The model under review builds one solid part; all positions refer to its coordinate system, in mm. Coordinates: 2 decimals unless noted, no trailing zeros. Write each loop counter-clockwise with the first axis right and the second up, starting at its lowest first coordinate (ties: lowest second). Pieces come first, ordered by that corner, then holes.
1) Add section C-C, the plane x = 31.75. State the section outline as (y, z) points (3 decimals), then the cut area to 3 significant figures.
2) Add section D-D, the plane z = 7. State the section outline as (x, y) points (3 decimals), then the cut area to 3 significant figures.
3) Add section B-B, the plane z = 20. State the section outline as (x, y) points (3 decimals).
4) Add section A-A, the plane z = 44.45. State the section outline as (x, y) points (3 decimals), then the cut area to 3 significant figures.
5) For line 1 (X direction, y = 2.5, z = 33.15); line 2 (X direction, y = 0.9, z = 44.45); line 3 (Z direction, x = 29, y = 0.4), list the stretches that pass through material, from the lowest coordinate up.
from build123d import *

# Parameters (mm, degrees)
SKETCH1_W          = 38.1
SKETCH1_H          = 50.8
SKETCH1_R          = 1.65
SKETCH1_R_2        = 7.5
SKETCH1_R_3        = 3.2639
BASE_EXTRUDE_DEPTH = 3.175


with BuildPart() as part:
    # Sketch1 → Base Extrude (new body)
    with BuildSketch(Plane(origin=(0, 0, 0), x_dir=(1, 0, 0), z_dir=(0, 1, 0))):
        with Locations((19.05, -25.4)):
            Rectangle(SKETCH1_W, SKETCH1_H)
        with Locations((19.05, -40.9)):
            Circle(SKETCH1_R, mode=Mode.SUBTRACT)
        with Locations((5.626606241, -33.15)):
            Circle(SKETCH1_R, mode=Mode.SUBTRACT)
        with Locations((5.626606241, -17.65)):
            Circle(SKETCH1_R, mode=Mode.SUBTRACT)
        with Locations((19.05, -9.9)):
            Circle(SKETCH1_R, mode=Mode.SUBTRACT)
        with Locations((32.473393759, -17.65)):
            Circle(SKETCH1_R, mode=Mode.SUBTRACT)
        with Locations((32.473393759, -33.15)):
            Circle(SKETCH1_R, mode=Mode.SUBTRACT)
        with Locations((19.05, -25.4)):
            Circle(SKETCH1_R_2, mode=Mode.SUBTRACT)
        with Locations((6.35, -6.35)):
            Circle(SKETCH1_R_3, mode=Mode.SUBTRACT)
        with Locations((31.75, -6.35)):
            Circle(SKETCH1_R_3, mode=Mode.SUBTRACT)
        with Locations((6.35, -44.45)):
            Circle(SKETCH1_R_3, mode=Mode.SUBTRACT)
        with Locations((31.75, -44.45)):
            Circle(SKETCH1_R_3, mode=Mode.SUBTRACT)
    extrude(amount=BASE_EXTRUDE_DEPTH)


solid = part.part
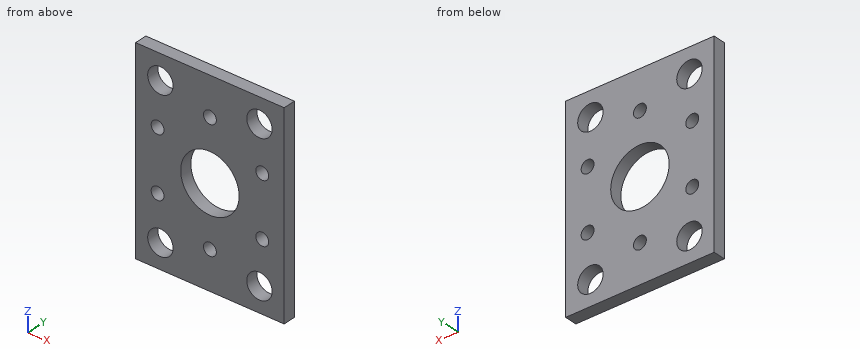
Geometry results:
1. outline: (0, 0) - (3.175, 0) - (3.175, 3.086) - (0, 3.086) - close; (0, 9.614) - (3.175, 9.614) - (3.175, 16.167) - (0, 16.167) - close; (0, 19.133) - (3.175, 19.133) - (3.175, 31.667) - (0, 31.667) - close; (0, 34.633) - (3.175, 34.633) - (3.175, 41.186) - (0, 41.186) - close; (0, 47.714) - (3.175, 47.714) - (3.175, 50.8) - (0, 50.8) - close
1. area: 101 mm2
2. outline: (0, 0) - (3.151, 0) - (3.151, 3.175) - (0, 3.175) - close; (9.549, 0) - (28.551, 0) - (28.551, 3.175) - (9.549, 3.175) - close; (34.949, 0) - (38.1, 0) - (38.1, 3.175) - (34.949, 3.175) - close
2. area: 80.3 mm2
3. outline: (0, 0) - (13.845, 0) - (13.845, 3.175) - (0, 3.175) - close; (24.255, 0) - (38.1, 0) - (38.1, 3.175) - (24.255, 3.175) - close
4. outline: (0, 0) - (3.086, 0) - (3.086, 3.175) - (0, 3.175) - close; (9.614, 0) - (28.486, 0) - (28.486, 3.175) - (9.614, 3.175) - close; (35.014, 0) - (38.1, 0) - (38.1, 3.175) - (35.014, 3.175) - close
4. area: 79.5 mm2
5. line 1: x = 0 to 3.98, 7.28 to 30.82, 34.12 to 38.1
5. line 2: x = 0 to 3.09, 9.61 to 28.49, 35.01 to 38.1
5. line 3: z = 0 to 4.59, 8.11 to 42.69, 46.21 to 50.8
